```python
from build123d import *

# Parameters (mm, degrees)
F0_W     = 30
F0_H     = 20
F1_DEPTH = 10
F3_D     = 8
F3_DEPTH = 50
F4_R     = 5


with BuildPart() as f1:
    # F0 (on Right) → F1 (new body, symmetric)
    with BuildSketch(Plane.YZ):
        with Locations((-15, 10)):
            Rectangle(F0_W, F0_H)
    extrude(amount=F1_DEPTH, both=True)

    # F3
    with Locations(Plane.XZ.offset(30)):
        with Locations((0, 10)):
            Hole(F3_D / 2, depth=F3_DEPTH)

    # F4
    f4_edges = [f1.edges().sort_by_distance(p)[0] for p in [
        (0, 0, 20),
        (0, -30, 20),
        (-10, -15, 20),
        (10, -15, 20),
        (10, -30, 10),
        (-10, -30, 10),
        (10, 0, 10),
        (-10, 0, 10),
    ]]
    fillet(f4_edges, radius=F4_R)


solid = f1.part
```
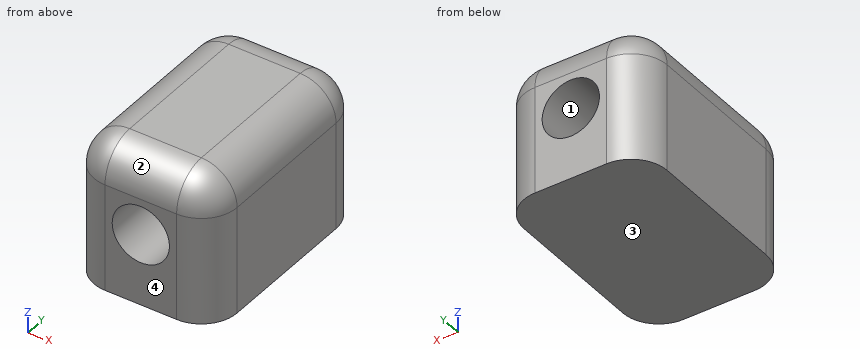
Read the model definition and answer for the solid it produces. Units are mm, in the model's axes. Face numbers are marked on the shaded views. Coordinates: 2 decimals unless noted, no trailing zeros. Loops run counter-clockwise (first coordinate to the right, second up) from the corner with the lowest first, then second, coordinate; pieces in that order, holes last. Notation, with made-up numbers: (-15.75, 73) - (6.25, 73) arc R4 cw to (6.25, 78) - close; hole circle Ø6 at (61, -4). An arc over 180 degrees is marked (long way). Answer in a Markdown table with one row per item.
1. Find section A-A, the plane y = -10. Write down the section's boundary in (x, z), then the cut area to 3 significant figures.
Conclusion:
| item | result |
|---|---|
| outline | (-10, 0) - (10, 0) - (10, 15) arc R5 ccw to (5, 20) - (-5, 20) arc R5 ccw to (-10, 15) - close; hole circle Ø8 at (0, 10) |
| area | 339 mm² |
2. Straight lines are drawn through the part: line 1 (Z direction, x = 0, y = -13.5); line 2 (Y direction, x = 5.25, z = 13.75); line 3 (X direction, y = -19.5, z = 10.5). For each, find the intervals that lie inside material, in ascending order.
Conclusion:
| item | result |
|---|---|
| line 1 | z = 0 to 6, 14 to 20 |
| line 2 | y = -29.99 to -0.01 |
| line 3 | x = -10 to -3.97, 3.97 to 10 |
3. Given pin 1 (6.5 mm diameter, centred on x = 0, z = 10, fed in from -Y) (1 decimal); pin 2 (1 mm diameter, centred on x = 7.5, y = -3.5, fed in from +Z), each flat-ended and moving along its own axis, determine where each tip first touches the part or whether it passes through.
Conclusion:
| item | result |
|---|---|
| pin 1 | passes through |
| pin 2 | stops at z = 19.38 |
4. Find section C-C, the plane z = 10. Write down the section's boundary in (x, y), then the cut area to 3 significant figures.
Conclusion:
| item | result |
|---|---|
| outline | (-10, -25) arc R5 ccw to (-5, -30) - (-4, -30) - (-4, 0) - (-5, 0) arc R5 ccw to (-10, -5) - close; (4, -30) - (5, -30) arc R5 ccw to (10, -25) - (10, -5) arc R5 ccw to (5, 0) - (4, 0) - close |
| area | 339 mm² |
5. Find section D-D, the plane z = 3.5. Write down the section's boundary in (x, y).
Conclusion:
| item | result |
|---|---|
| outline | (-10, -25) arc R5 ccw to (-5, -30) - (5, -30) arc R5 ccw to (10, -25) - (10, -5) arc R5 ccw to (5, 0) - (-5, 0) arc R5 ccw to (-10, -5) - close |
6. Determine the mould class of the marked faces 1, 2, 3 and 4 for opening direction Z: +Z half, -Z half, draft (parallel to the pull), parting line (faces both ways), or undercut.
Conclusion:
| item | result |
|---|---|
| face 1 | undercut |
| face 2 | +Z half |
| face 3 | -Z half |
| face 4 | draft |
7. Find section B-B, the plane x = 0. Write down the section's boundary in (y, z).
Conclusion:
| item | result |
|---|---|
| outline | (-30, 0) - (0, 0) - (0, 6) - (-30, 6) - close; (-30, 14) - (0, 14) - (0, 15) arc R5 ccw to (-5, 20) - (-25, 20) arc R5 ccw to (-30, 15) - close |
